Build history of the part. All positions in model axes, mm. A direction names the side the tool comes from. Give positions to 0.01 mm unless a question says otherwise; leave off trailing zeros. Loops run counter-clockwise (first coordinate to the right, second up) from the corner with the lowest first, then second, coordinate; pieces in that order, holes last. Notation, with made-up numbers: (16.5, -31.75) -> (75.5, -31.75) arc R33 ccw to (75.5, 7.25) -> close; hole circle Ø3 at (86, 23). An arc over 180 degrees is marked (long way). Answer as a JSON object with one key per item and string values. Group by question number.
Q1. Band-saw the part on B-B, the plane y = 14.5. Write the cut outline in (x, z).
Q2. Two-plate mould, pull along Y, no slides. Class faces 1 (the flat face through (23, 25.4, 246)), 2 (the flat face through (11.588, 13, 246)), 3 (the flat face through (35.4, 13, 246)): pulls with the +Y half, pulls with the -Y half, needs draft (parallel to the pull), parting line crosses it, or undercut.
Q3. Band-saw the part on A-A, the plane x = 16. Write the cut outline in (y, z).
Q4. Wall check: probe 1 along X at (y, z) = (22, 355.5); probe 2 along Y at (x, z) = (28.25, 110). Give the ranges that are in metal, low to high. Write a range as from..to.
Q5. Drop a flat-ended pin along its axis: pin 1 (5 mm diameter, centred on x = 21.5, y = 5, fed in from -Z). Give the stop position or say it passes through.
Q6. Tool access for faces 4 (the flat face through (23, 1.588, 246)), 5 (the flat face through (23, 0, 246)): list every direction of +Z, -Z, +X, -X, +Y, -Y with a clear straight run to the whole face (end or side of a thin tool).
Q7. Band-saw the part on C-C, the plane z = 274.5. Write the cut outline in (x, y), plus the area to 3 significant figures.
Autodesk Inventor part; units mm, degrees
ref_plane "YZ Plane" through (0, 0, 0) normal (1, 0, 0) x (0, 1, 0)
ref_plane "XZ Plane" through (0, 0, 0) normal (0, 1, 0) x (-1, 0, 0)
ref_plane "XY Plane" through (0, 0, 0) normal (0, 0, 1) x (1, 0, 0)
sketch "Sketch1" plane through (0, 0, 0) normal (0, 0, 1) x (1, 0, 0)
  line L0 (93.1, 0) -> (67.7, 0)
  line L1 (93.1, 0) -> (67.7, 0)
  line L2 (10, 0) -> (35.4, 0)
  line L3 (35.4, 0) -> (35.4, 25.4)
  line L4 (35.4, 25.4) -> (10, 25.4)
  line L5 (10, 25.4) -> (10, 0)
  line L6 (11.5875, 1.5875) -> (33.8125, 1.5875)
  line L7 (33.8125, 1.5875) -> (33.8125, 23.8125)
  line L8 (33.8125, 23.8125) -> (11.5875, 23.8125)
  line L9 (11.5875, 23.8125) -> (11.5875, 1.5875)
  line L10 (67.7, 25.4) -> (67.7, 0)
  line L11 (93.1, 0) -> (93.1, 25.4)
  line L12 (93.1, 25.4) -> (67.7, 25.4)
  line L13 (67.7, 25.4) -> (67.7, 0)
  line L14 (93.1, 0) -> (93.1, 25.4)
  line L15 (93.1, 25.4) -> (67.7, 25.4)
  point P0 (0, 0)
  dimension "d0" = 22.225
  dimension "d1" = 22.225
  dimension "d3" = 1.5875
extrude "Extrusion1" add sketch "Sketch1" along normal blind 500 contours L5 L4 L3 L2
properties part number "LateralBars"
Worked answers:
{
 "1": {"outline": "(10, 0) -> (11.59, 0) -> (11.59, 500) -> (10, 500) -> close; (33.81, 0) -> (35.4, 0) -> (35.4, 500) -> (33.81, 500) -> close"},
 "2": {"face 1": "pulls with the +Y half", "face 2": "undercut", "face 3": "needs draft"},
 "3": {"outline": "(0, 0) -> (1.59, 0) -> (1.59, 500) -> (0, 500) -> close; (23.81, 0) -> (25.4, 0) -> (25.4, 500) -> (23.81, 500) -> close"},
 "4": {"probe 1": "10..11.59, 33.81..35.4", "probe 2": "0..1.59, 23.81..25.4"},
 "5": {"pin 1": "through"},
 "6": {"face 4": "+Z, -Z", "face 5": "+Z, -Z, +X, -X, -Y"},
 "7": {"outline": "(10, 0) -> (35.4, 0) -> (35.4, 25.4) -> (10, 25.4) -> close; hole (11.59, 1.59) -> (33.81, 1.59) -> (33.81, 23.81) -> (11.59, 23.81) -> close", "area": "151 mm2"}
}
